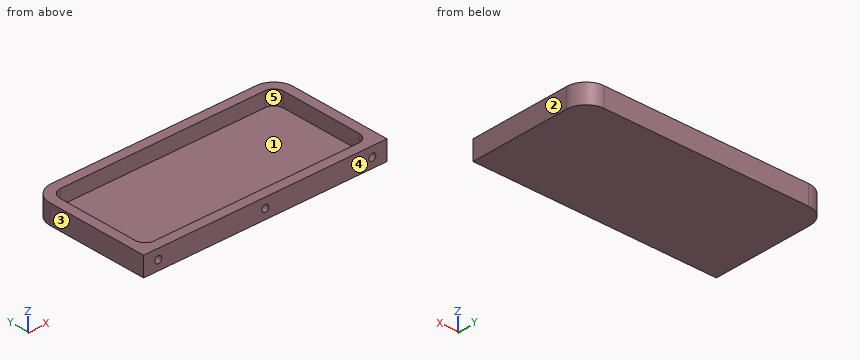
from build123d import *

# Parameters (mm, degrees)
SKETCH1_W                 = 79.375
SKETCH1_H                 = 39.37
BOSS_EXTRUDE1_DEPTH       = 6.35
FILLET1_R                 = 6.35
F_4_40_TAPPED_HOLE1_D     = 2.2606
F_4_40_TAPPED_HOLE1_DEPTH = 7.62
F_4_40_TAPPED_HOLE1_TIP   = 0.679152758
CUT_EXTRUDE1_DEPTH        = 4.7625


with BuildPart() as part:
    # Sketch1 → Boss-Extrude1 (new body)
    with BuildSketch(Plane.XY):
        Rectangle(SKETCH1_W, SKETCH1_H)
    extrude(amount=BOSS_EXTRUDE1_DEPTH)

    # Fillet1
    fillet1_edges = [part.edges().sort_by_distance(p)[0] for p in [
        (-39.6875, 19.685, 3.175),
        (39.6875, 19.685, 3.175),
    ]]
    fillet(fillet1_edges, radius=FILLET1_R)

    # #4-40 Tapped Hole1
    with Locations(Plane.XZ.offset(19.685)):
        with Locations((0, 3.175), (-34.925, 3.175), (34.925, 3.175)):
            Hole(F_4_40_TAPPED_HOLE1_D / 2, depth=F_4_40_TAPPED_HOLE1_DEPTH)
            with Locations((0, 0, -(F_4_40_TAPPED_HOLE1_DEPTH + F_4_40_TAPPED_HOLE1_TIP / 2))):  # 118° drill point
                Cone(0, F_4_40_TAPPED_HOLE1_D / 2, F_4_40_TAPPED_HOLE1_TIP, mode=Mode.SUBTRACT)

    # Sketch5 → Cut-Extrude1 (cut)
    with BuildSketch(Plane.XY.offset(6.35)):
        with BuildLine():
            Line((36.5125, -13.335), (36.5125, 13.335))
            ThreePointArc((36.5125, 13.335), (35.58256403, 15.58006403), (33.3375, 16.51))
            Line((33.3375, 16.51), (-33.3375, 16.51))
            ThreePointArc((-33.3375, 16.51), (-35.58256403, 15.58006403), (-36.5125, 13.335))
            Line((-36.5125, 13.335), (-36.5125, -13.335))
            ThreePointArc((-36.5125, -13.335), (-35.58256403, -15.58006403), (-33.3375, -16.51))
            Line((-33.3375, -16.51), (33.3375, -16.51))
            ThreePointArc((33.3375, -16.51), (35.58256403, -15.58006403), (36.5125, -13.335))
        make_face()
    extrude(amount=-CUT_EXTRUDE1_DEPTH, mode=Mode.SUBTRACT)


solid = part.part
Work out the finished part from the listing and answer in its coordinate system (mm). Face numbers are marked on the shaded views. A direction names the side the tool comes from. Coordinates: 2 decimals unless noted, no trailing zeros. Loops run counter-clockwise (first coordinate to the right, second up) from the corner with the lowest first, then second, coordinate; pieces in that order, holes last. Notation, with made-up numbers: M 4,45.5 L 50,45.5 A26 cw 50,73.5 Z; hole C -31,56 d5. An arc over 180 degrees is marked long. Answer in a Markdown table with one row per item. Add a question column.
1. The mould has two halves that part along Y. Classify the marked faces 3, 4 and 5: pulls with the +Y half, pulls with the -Y half, needs draft (parallel to the pull), parting line crosses it, or undercut.
2. Find section B-B, the plane y = 8.5. Write down the section's boundary in (x, z).
3. Flat-ended cylindrical pins translate along their axes: P1, Ø1.8, axis at x = -34.925, z = 3.175, coming from the +Y side; P2, Ø10, axis at x = -9, y = 1.5, coming from the +Z side. Find the tip coordinate at first contact, or state that the pin passes through.
4. A tool of negligible diameter and unlimited length cuts with its end or side. For the marked faces 1 and 2, from which of +Z, -Z, +X, -X, +Y, -Y can it reach the whole face along a straight path? Write none if from no direction.
5. Consider L1, parallel to X at y = 13.5, z = 3.25; L2, parallel to Y at x = 29, z = 6 (3 decimals); L3, parallel to Z at x = 0, y = -17. Determine where each line is inside the solid, lowest interval first.
Reported:
| question | item | result |
|---|---|---|
| 1 | face 3 | needs draft |
| 1 | face 4 | pulls with the -Y half |
| 1 | face 5 | undercut |
| 2 | outline | M -39.69,0 L 39.69,0 L 39.69,6.35 L 36.51,6.35 L 36.51,1.59 L -36.51,1.59 L -36.51,6.35 L -39.69,6.35 Z |
| 3 | P1 | stops at y = 19.65 |
| 3 | P2 | stops at z = 1.59 |
| 4 | face 1 | +Z |
| 4 | face 2 | +Z, -Z, +X, +Y, -Y |
| 5 | L1 | x = -39.69 to -36.51, 36.51 to 39.69 |
| 5 | L2 | y = -19.685 to -16.51, 16.51 to 19.685 |
| 5 | L3 | z = 0 to 2.04, 4.31 to 6.35 |
